Read the model definition and answer for the solid it produces. Units are mm, in the model's axes. Face numbers are marked on the shaded views. A direction names the side the tool comes from. Round coordinates to 2 decimals unless told otherwise and drop trailing zeros. Order: outer loops, then holes, each group sorted by start corner. A loop starts at its lowest first (then second) coordinate and runs counter-clockwise, first axis right, second up. Notation, with made-up numbers: (-20.75, 16.5) -> (-15.75, 16.5) arc R23 cw to (-15.75, 35.5) -> close; hole circle Ø9 at (-31.5, -9.75). An arc over 180 degrees is marked (long way). Use a Markdown table: item, result. Add a question column.
1. For the marked faces 4, 5 and 6, determine the directions among +Z, -Z, +X, -X, +Y, -Y from which every point of the face is accessible in a straight line to the end or side of a thin tool.
2. Section B-B, the plane y = 24 is taken. Give the vertices of the cut face in (x, z).
3. Section C-C, the plane z = 16.5 is taken. Give the vertices of the cut face in (x, y).
4. Section A-A, the plane x = 45.5 is taken. Give the vertices of the cut face in (y, z).
5. Consider L1, parallel to Y at x = 44, z = 13.5; L2, parallel to X at y = 21, z = 24.5; L3, parallel to X at y = 21.5, z = 30. Determine where each line is inside the solid, lowest interval first. Write a range as [from, to].
6. Given pin 1 (1.5 mm diameter, centred on x = 15, z = 44.5, fed in from -Y); pin 2 (1.5 mm diameter, centred on x = 19, z = 25, fed in from +Y); pin 3 (6 mm diameter, centred on x = 41, y = 18.5, fed in from +Z); pin 4 (11 mm diameter, centred on y = 44.5, z = 14, fed in from -X), each flat-ended and moving along its own axis, determine where each tip first touches the part or whether it passes through.
7. The mould has two halves that part along Y. Classify the marked faces 1, 2 and 3: +Y half, -Y half, draft (parallel to the pull), parting line (faces both ways), or undercut.
8. Section D-D, the plane y = 9 is taken. Give the vertices of the cut face in (x, z).
```python
from build123d import *

# Parameters (mm, degrees)
BOSS_EXTRUDE1_DEPTH = 50
SKETCH2_W           = 20
SKETCH2_H           = 20
CUT_EXTRUDE1_DEPTH  = 20
CUT_EXTRUDE2_DEPTH  = 10
SKETCH4_W           = 50
SKETCH4_H           = 10
BOSS_EXTRUDE2_DEPTH = 50
SKETCH5_W           = 50
SKETCH5_H           = 10
CUT_EXTRUDE5_DEPTH  = 30
SKETCH6_W           = 20
SKETCH6_H           = 20
BOSS_EXTRUDE4_DEPTH = 5
CUT_EXTRUDE8_DEPTH  = 40
CUT_EXTRUDE9_DEPTH  = 70


with BuildPart() as part:
    # Sketch1 → Boss-Extrude1 (new body)
    with BuildSketch(Plane.XY):
        Polygon((0, 0), (0, 20), (20, 40), (70, 40), (70, 0), align=None)
    extrude(amount=BOSS_EXTRUDE1_DEPTH)

    # Sketch2 → Cut-Extrude1 (cut)
    with BuildSketch(Plane.XY.offset(50)):
        with Locations((40, 10)):
            Rectangle(SKETCH2_W, SKETCH2_H)
    extrude(amount=-CUT_EXTRUDE1_DEPTH, mode=Mode.SUBTRACT)

    # Sketch3 → Cut-Extrude2 (cut)
    with BuildSketch(Plane.XY.offset(50)):
        Polygon((30, 20), (40, 40), (60, 40), (50, 20), align=None)
    extrude(amount=-CUT_EXTRUDE2_DEPTH, mode=Mode.SUBTRACT)

    # Sketch4 → Boss-Extrude2 (add)
    with BuildSketch(Plane.XY.offset(50)):
        with Locations((45, 45)):
            Rectangle(SKETCH4_W, SKETCH4_H)
    extrude(amount=-BOSS_EXTRUDE2_DEPTH)

    # Sketch5 → Cut-Extrude5 (cut)
    with BuildSketch(Plane.XY.offset(50)):
        with Locations((45, 45)):
            Rectangle(SKETCH5_W, SKETCH5_H)
    extrude(amount=-CUT_EXTRUDE5_DEPTH, mode=Mode.SUBTRACT)

    # Sketch6 → Boss-Extrude4 (add)
    with BuildSketch(Plane.XY.offset(30)):
        with Locations((40, 10)):
            Rectangle(SKETCH6_W, SKETCH6_H)
    extrude(amount=BOSS_EXTRUDE4_DEPTH)

    # Sketch8 → Cut-Extrude8 (cut)
    with BuildSketch(Plane.XY.offset(40)):
        Polygon((40, 40), (60, 40), (50, 20), (30, 20), align=None)
    extrude(amount=-CUT_EXTRUDE8_DEPTH, mode=Mode.SUBTRACT)

    # Sketch9 → Cut-Extrude9 (cut)
    with BuildSketch(Plane.ZY):
        Polygon((20, 40), (35, 20), (50, 20), (50, 40), align=None)
        Polygon((35, 20), (50, 0), (50, 20), align=None)
    extrude(amount=-CUT_EXTRUDE9_DEPTH, mode=Mode.SUBTRACT)


solid = part.part
```
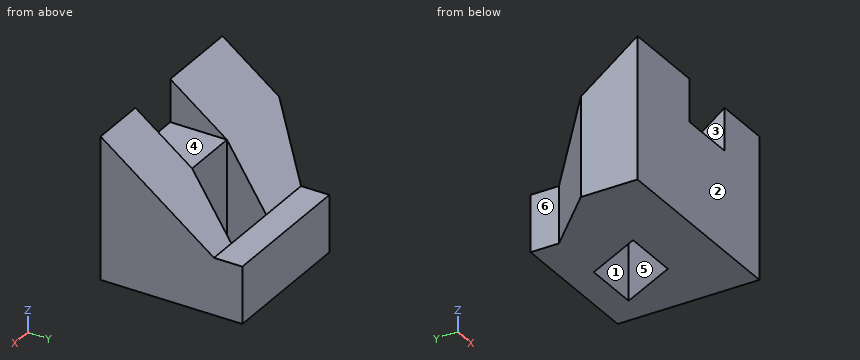
Verdict:
| question | item | result |
|---|---|---|
| 1 | face 4 | +Z, +Y, -Y |
| 1 | face 5 | +Z, -Z |
| 1 | face 6 | +Z, -Z, -X, +Y |
| 2 | outline | (4, 0) -> (32, 0) -> (32, 32) -> (4, 32) -> close; (52, 0) -> (70, 0) -> (70, 32) -> (52, 32) -> close |
| 3 | outline | (0, 0) -> (70, 0) -> (70, 50) -> (20, 50) -> (20, 40) -> (0, 20) -> close; hole (30, 20) -> (50, 20) -> (60, 40) -> (40, 40) -> close |
| 4 | outline | (0, 0) -> (20, 0) -> (20, 35) -> (0, 35) -> close; (40, 0) -> (50, 0) -> (50, 20) -> (40, 20) -> close |
| 5 | L1 | y = [0, 20], [40, 50] |
| 5 | L2 | x = [1, 30.5], [50.5, 70] |
| 5 | L3 | x = [1.5, 30.75], [50.75, 70] |
| 6 | pin 1 | stops at y = 0 |
| 6 | pin 2 | stops at y = 34.33 |
| 6 | pin 3 | stops at z = 35 |
| 6 | pin 4 | stops at x = 19 |
| 7 | face 1 | undercut |
| 7 | face 2 | -Y half |
| 7 | face 3 | draft |
| 8 | outline | (0, 0) -> (70, 0) -> (70, 43.25) -> (50, 43.25) -> (50, 35) -> (30, 35) -> (30, 43.25) -> (0, 43.25) -> close |
